For this review, take the finished solid that the model builds, in its own axes (mm). Face numbers are marked on the shaded views. Coordinates: 2 decimals unless noted, no trailing zeros. Order: outer loops, then holes, each group sorted by start corner. A loop starts at its lowest first (then second) coordinate and runs counter-clockwise, first axis right, second up. Notation, with made-up numbers: (14, -2.5) -> (50, -2.5) arc R7 cw to (50, 2.5) -> close; hole circle Ø3 at (-2.75, 82.5). An arc over 180 degrees is marked (long way). Write item = value, one per line. Start each with the question number.
1) Insertion check: pin 1 Ø16.5 at (x, z) = (-34.5, 43) entering from -Y; pin 2 Ø2 at (x, y) = (-8, 0.5) entering from +Z; pin 3 Ø3.5 at (x, y) = (-30.5, 2.5) entering from -Z. Each pin has a flat end and moves straight along its axis. Give the tip position at first contact, or say it passes through.
2) Consider section A-A on z = 0. Give the boundary of the cut face in (x, y), and give its area (3 significant figures).
3) Consider section C-C on z = 22. Give the boundary of the cut face in (x, y).
4) Draft analysis for pull direction Z (two halves, no side actions). For the marked faces 1 and 2, state which applies: +Z half, -Z half, draft (parallel to the pull), parting line (faces both ways), or undercut.
5) Wall thickness on probe 1 along Y at (x, z) = (-54, 0); probe 2 along Y at (x, z) = (-64.5, 26); probe 3 along X at (y, z) = (1.25, 1): over which ranges is each line inside the solid? List them lowest first. Write a range as [from, to].
from build123d import *

# Parameters (mm, degrees)
SKETCH2_R           = 1.1
BOSS_EXTRUDE1_DEPTH = 80
CUT_EXTRUDE1_START  = 40
CUT_EXTRUDE1_DEPTH  = 11
CUT_EXTRUDE2_DEPTH  = 101.797135376
FILLET1_R           = 0.5


with BuildPart() as part:
    # Sketch2 → Boss-Extrude1 (new body)
    with BuildSketch(Plane(origin=(0, 0, 0), x_dir=(0, 0, -1), z_dir=(1, 0, 0))):
        with BuildLine():
            ThreePointArc((-2.015564437, -1), (2.25, 0), (-2.015564437, 1))
            Line((-2.015564437, 1), (-56, 1))
            Line((-56, 1), (-56, 4))
            Line((-56, 4), (-61, 4))
            Line((-61, 4), (-61, 3))
            Line((-61, 3), (-57, 3))
            Line((-57, 3), (-57, 1))
            Line((-57, 1), (-57, -1))
            Line((-57, -1), (-2.015564437, -1))
        make_face()
        Circle(SKETCH2_R, mode=Mode.SUBTRACT)
    extrude(amount=-BOSS_EXTRUDE1_DEPTH)

    # Sketch5 → Cut-Extrude1 (cut)
    with BuildSketch(Plane(origin=(-40, 0, 0), x_dir=(0, 0, -1), z_dir=(1, 0, 0)).offset(CUT_EXTRUDE1_START)):
        with BuildLine():
            Line((-2.015564437, 1), (-5.015564437, 1))
            Line((-5.015564437, 1), (-5.015564437, -1))
            Line((-5.015564437, -1), (-2.015564437, -1))
            ThreePointArc((-2.015564437, -1), (2.25, 0), (-2.015564437, 1))
        make_face()
    cut_extrude1 = extrude(amount=-CUT_EXTRUDE1_DEPTH, mode=Mode.SUBTRACT)

    # Mirror1: Cut-Extrude1 across plane
    add(cut_extrude1.mirror(Plane(origin=(-40, 0, 0), x_dir=(0, 0, 1), z_dir=(1, 0, 0))), mode=Mode.SUBTRACT)

    # Sketch6 → Cut-Extrude2 (cut, through all)
    with BuildSketch(Plane(origin=(0, 4, 0), x_dir=(1, 0, 0), z_dir=(0, 1, 0))):
        Polygon((-65, -56), (-60, -61), (-80, -61), (-80, -56), align=None)
        Polygon((-15, -56), (-20, -61), (0, -61), (0, -56), align=None)
    extrude(amount=-CUT_EXTRUDE2_DEPTH, mode=Mode.SUBTRACT)

    # Fillet1
    fillet1_edges = [part.edges().sort_by_distance(p)[0] for p in [
        (-17.5, 4, 58.5),
        (-62.5, 4, 58.5),
        (-40, 4, 61),
        (0, 0, 5.015564437),
        (0, 0, 56),
        (-80, 0, 5.015564437),
        (-80, 0, 56),
        (-40, 3, 61),
        (-16, 1, 57),
        (-64, 1, 57),
        (-72.5, 1, 56),
        (-7.5, 1, 56),
        (0, 1, 30.507782219),
        (-80, 1, 30.507782219),
    ]]
    fillet(fillet1_edges, radius=FILLET1_R - 0.0001)  # a hair under: the kernel refuses the full size


solid = part.part
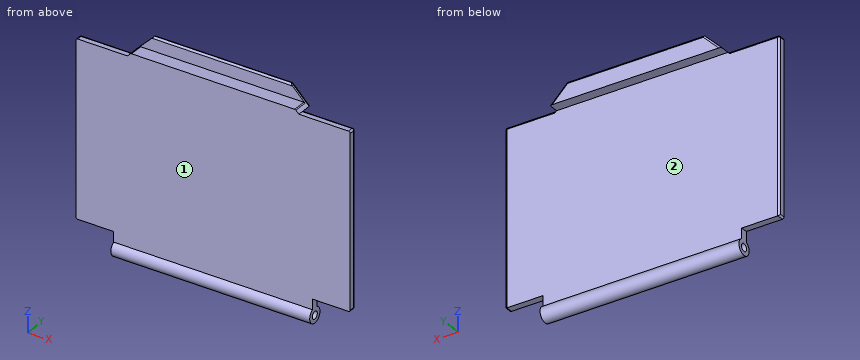
Answer sheet:
q1.pin_1 = -1
q1.pin_2 = 56
q1.pin_3 = -2.12
q2.outline = (-69, -2.25) -> (-11, -2.25) -> (-11, -1.1) -> (-69, -1.1) -> close; (-69, 1.1) -> (-11, 1.1) -> (-11, 2.25) -> (-69, 2.25) -> close
q2.area = 133 mm2
q3.outline = (-80, -1) -> (0, -1) -> (0, 0.5) arc R0.5 ccw to (-0.5, 1) -> (-79.5, 1) arc R0.5 ccw to (-80, 0.5) -> close
q4.face_1 = draft
q4.face_2 = undercut
q5.probe_1 = [-2.25, -1.1], [1.1, 2.25]
q5.probe_2 = [-1, 1]
q5.probe_3 = [-69, -11]
